from build123d import *

# Parameters (mm, degrees)
BOSS_EXTRUDE1_DEPTH     = 4
CUT_EXTRUDE1_DEPTH      = 10
CUT_EXTRUDE1_DEPTH_BACK = 10
SKETCH4_W               = 4
SKETCH4_H               = 50.01485274
BOSS_EXTRUDE3_DEPTH     = 2.69


with BuildPart() as part:
    # Sketch2 → Boss-Extrude1 (new body)
    with BuildSketch(Plane(origin=(0, 0, 0), x_dir=(0, 0, -1), z_dir=(1, 0, 0))):
        Polygon((61, 4), (101, 4), (101, 0), (161.781661072, 0), (161.781661072, -10), (165.781661072, -10), (165.781661072, -37), (161.781661072, -37), (161.781661072, -46.015400021), (1, -46.015400021), (1, -37), (-3, -37), (-3, -10), (1, -10), (1, 0), (61, 0), align=None)
    extrude(amount=BOSS_EXTRUDE1_DEPTH)

    # Sketch3 → Cut-Extrude1 (cut, two sides)
    with BuildSketch(Plane(origin=(0, 0, 0), x_dir=(0, 0, -1), z_dir=(1, 0, 0))) as cut_extrude1_sk:
        Polygon((77, 4.594080923), (187.139354616, 4.594080923), (187.139354616, -56.777475016), (77, -56.777475016), (77, -46.986682045), align=None)
    extrude(amount=CUT_EXTRUDE1_DEPTH, mode=Mode.SUBTRACT)
    extrude(cut_extrude1_sk.sketch, amount=-CUT_EXTRUDE1_DEPTH_BACK, mode=Mode.SUBTRACT)

    # Sketch4 → Boss-Extrude3 (add)
    with BuildSketch(Plane(origin=(0, 0, -77), x_dir=(-1, 0, 0), z_dir=(0, 0, -1))):
        with Locations((-2, -21.007973651)):
            Rectangle(SKETCH4_W, SKETCH4_H)
    extrude(amount=BOSS_EXTRUDE3_DEPTH)


solid = part.part
Geometry: final body of the model. Coordinates: model frame, mm. A direction names the side the tool comes from. Coordinates: 2 decimals unless noted, no trailing zeros. Loops run counter-clockwise (first coordinate to the right, second up) from the corner with the lowest first, then second, coordinate; pieces in that order, holes last. Notation, with made-up numbers: M 68.25,26.25 L 76.25,26.25 A5 ccw 76.25,35.25 Z; hole C 45.25,31.25 d4. An arc over 180 degrees is marked long. One line per item, written item: value. Start each with the question number.
1) Cut plane B-B (z = -2). Return loops of the section in (x, y), then the cut area to 3 significant figures.
2) Pin query (flat end, axial travel): P1, Ø2, axis at x = 3, z = 0.5, coming from the +Y side; P2, Ø1.2, axis at x = 1.5, z = 1, coming from the -Y side; P3, Ø1.5, axis at x = 2.5, z = -33.5, coming from the +Y side. Return the tip coordinate at first contact, or that it passes through.
3) Reachability of faces 1 (the flat face through (2, -37, 1)), 2 (the flat face through (0, -21, -38)), 3 (the flat face through (2, -5, -1)) from +Z, -Z, +X, -X, +Y, -Y: full face, straight path, thin tool, end or side. Return the list, or none.
4) Material intervals for L1, parallel to Y at x = 2, z = -24.5; L2, parallel to Z at x = 2.4, y = -7, sorted ascending. Write a range as from..to.
Evaluation:
1. outline: M 0,-46.02 L 4,-46.02 L 4,0 L 0,0 Z
1. area: 184 mm^2
2. P1: y = -10
2. P2: y = -37
2. P3: y = 0
3. face 1: +Z, +X, -X, -Y
3. face 2: +Z, -Z, -X, +Y, -Y
3. face 3: +Z, +X, -X, +Y
4. L1: -46.02..0
4. L2: -79.69..-1
